```python
from build123d import *

# Parameters (mm, degrees)
F0_W     = 152.4
F0_H     = 127
F1_DEPTH = 381
F2_T     = -2.54
F3_W     = 162.56
F3_H     = 391.16
F3_W_2   = 152.4
F3_H_2   = 381
F4_DEPTH = 25.4


with BuildPart() as f1:
    # F0 (on Front) → F1 (new body)
    with BuildSketch(Plane.XZ):
        with Locations((76.2, 63.5)):
            Rectangle(F0_W, F0_H)
    extrude(amount=-F1_DEPTH)

    # F2
    f2_openings = [f1.faces().sort_by_distance(p)[0] for p in [
        (76.2, 190.5, 127),
    ]]
    offset(amount=F2_T, openings=f2_openings)

    # F3 (on face) → F4 (join)
    with BuildSketch(Plane.XY.offset(127)):
        with Locations((76.2, 190.5)):
            Rectangle(F3_W, F3_H)
        with Locations((76.2, 190.5)):
            Rectangle(F3_W_2, F3_H_2, mode=Mode.SUBTRACT)
    extrude(amount=-F4_DEPTH)


solid = f1.part
```
Read the model definition and answer for the solid it produces. Units are mm, in the model's axes. A direction names the side the tool comes from. Round coordinates to 2 decimals unless told otherwise and drop trailing zeros. Write each loop counter-clockwise with the first axis right and the second up, starting at its lowest first coordinate (ties: lowest second). Pieces come first, ordered by that corner, then holes. Notation, with made-up numbers: (58.25, 3.25) - (117.25, 3.25) arc R26 cw to (117.25, 18.25) - close; hole circle Ø11 at (75, 18). An arc over 180 degrees is marked (long way). Use CSV: the item, a comma, the result in double quotes.
Q1. Find section B-B, the plane y = 359. Write down the section's boundary in (x, z), then the cut area to 3 significant figures.
Values:
outline,"(-5.08, 101.6) - (0, 101.6) - (0, 0) - (152.4, 0) - (152.4, 101.6) - (157.48, 101.6) - (157.48, 127) - (149.86, 127) - (149.86, 2.54) - (2.54, 2.54) - (2.54, 127) - (-5.08, 127) - close"
area,"1,280 mm²"
Q2. Determine the mould class of faces 1 (the flat face through (149.86, 188, 64)), 2 (the flat face through (75, 381, 52)), 3 (the flat face through (157.48, 188, 114)) for opening direction X: +X half, -X half, draft (parallel to the pull), parting line (faces both ways), or undercut.
Values:
face 1,"undercut"
face 2,"draft"
face 3,"+X half"
Q3. Each of these flat-tipped pins is pushed along its axis until it touches: pin 1 Ø8 at (y, z) = (259.5, 65.5) entering from -X; pin 2 Ø12 at (y, z) = (335.5, 97.5) entering from +X; pin 3 Ø3 at (y, z) = (98.5, 35) entering from +X; pin 4 Ø8 at (x, z) = (52, 70.5) entering from +Y. Where does it stop, or does it pass through?
Values:
pin 1,"stops at x = 0"
pin 2,"stops at x = 157.48"
pin 3,"stops at x = 152.4"
pin 4,"stops at y = 381"
Q4. A tool of negligible diameter and unlimited length cuts with its end or side. For faces 4 (the flat face through (0, 188, 50)), 5 (the flat face through (75, 0, 52)), 6 (the flat face through (75, 378.46, 66)), 7 (the flat face through (-5.08, 188, 114)), 8 (the flat face through (152.4, 188, 50)), from which of +Z, -Z, +X, -X, +Y, -Y can it reach the whole face along a straight path? Write none if from no direction.
Values:
face 4,"-Z, -X, +Y, -Y"
face 5,"-Z, +X, -X, -Y"
face 6,"+Z"
face 7,"+Z, -Z, -X, +Y, -Y"
face 8,"-Z, +X, +Y, -Y"
Q5. Find section C-C, the plane x = 113. Write down the section's boundary in (y, z), then the cut area to 3 significant figures.
Values:
outline,"(-5.08, 101.6) - (0, 101.6) - (0, 0) - (381, 0) - (381, 101.6) - (386.08, 101.6) - (386.08, 127) - (378.46, 127) - (378.46, 2.54) - (2.54, 2.54) - (2.54, 127) - (-5.08, 127) - close"
area,"1,860 mm²"
Q6. Straight lines are drawn through the part: line 1 along X through (y, z) = (101, 9); line 2 along Y through (x, z) = (95.5, 9.5); line 3 along Y through (x, z) = (144.5, 117.5). For each, find the intervals that lie inside material, in ascending order.
Values:
line 1,"x = 0 to 2.54, 149.86 to 152.4"
line 2,"y = 0 to 2.54, 378.46 to 381"
line 3,"y = -5.08 to 2.54, 378.46 to 386.08"
Q7. Find section A-A, the plane z = 50. Write down the section's boundary in (x, y).
Values:
outline,"(0, 0) - (152.4, 0) - (152.4, 381) - (0, 381) - close; hole (2.54, 2.54) - (149.86, 2.54) - (149.86, 378.46) - (2.54, 378.46) - close"
